Study the drawing (mm; zero at the part's minimum x, y, z) and answer. A direction names the side the tool comes from. Give positions to 0.01 mm unless a question says otherwise; leave off trailing zeros. Loops run counter-clockwise (first coordinate to the right, second up) from the corner with the lowest first, then second, coordinate; pieces in that order, holes last. Notation, with made-up numbers: M 81,15.5 L 135,15.5 A26 cw 135,41.5 Z; hole C 43.5,-24.75 d10. An arc over 180 degrees is marked long. Return JSON: item names as keys, results as strings.
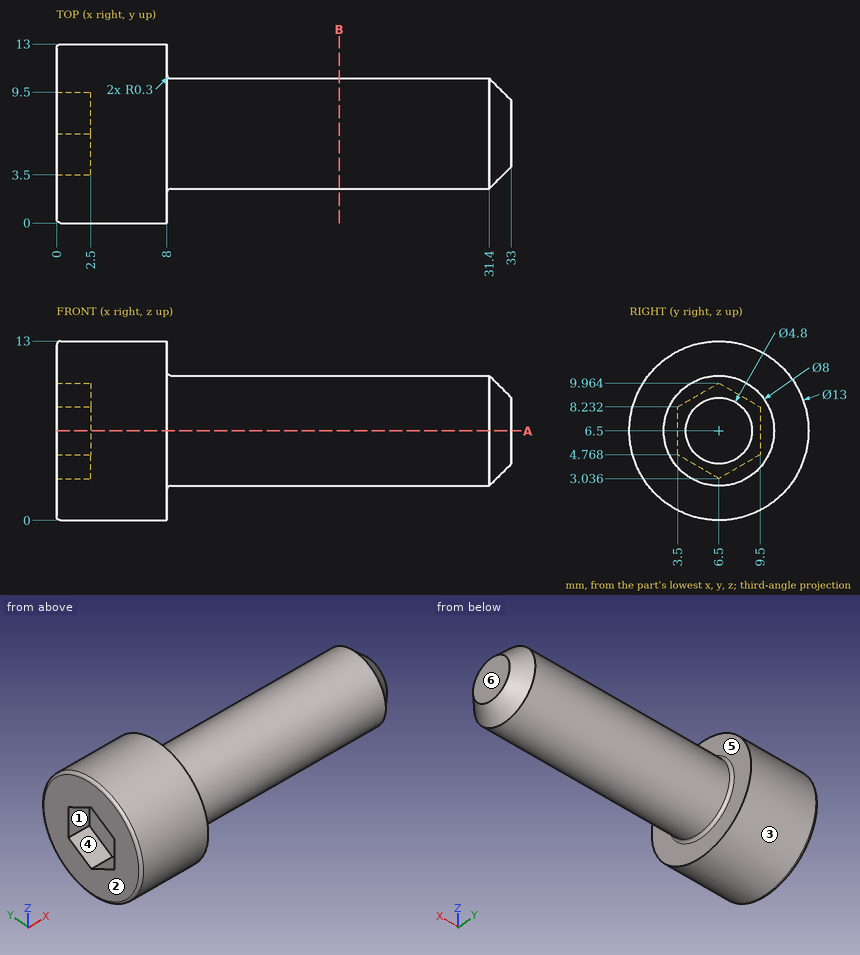
(1) Given pin 1 (2 mm diameter, centred on y = 6, z = 1.5, fed in from -X); pin 2 (1.5 mm diameter, centred on y = 9.5, z = 2.5, fed in from +X); pin 3 (1.8 mm diameter, centred on y = 7, z = 5, fed in from -X); pin 4 (4 mm diameter, centred on x = 29.5, y = 11.5, fed in from +Z), each flat-ended and moving along its own axis, determine where each tip first touches the part or whether it passes through.
Values follow:
{"pin 1": "x = 0", "pin 2": "x = 8", "pin 3": "x = 2.5", "pin 4": "z = 9.15"}
(2) The part is cut by section A-A (z = 6.5). Determine the outline of the cut face in (x, y).
Values follow:
{"outline": "M 0,0.3 A0.3 ccw 0.3,0 L 8,0 L 8,2.2 A0.3 cw 8.3,2.5 L 31.4,2.5 L 33,4.1 L 33,8.9 L 31.4,10.5 L 8.3,10.5 A0.3 cw 8,10.8 L 8,13 L 0.3,13 A0.3 ccw 0,12.7 L 0,9.5 L 2.5,9.5 L 2.5,3.5 L 0,3.5 Z"}
(3) Straight lines are drawn through the part: line 1 along Z through (x, y) = (18, 6.25); line 2 along Y through (x, z) = (13.5, 4.5); line 3 along X through (y, z) = (5.75, 6.75). For each, find the intervals that lie inside material, in ascending order.
Values follow:
{"line 1": "2.51 to 10.49", "line 2": "3.04 to 9.96", "line 3": "2.5 to 33"}
(4) The part is cut by section B-B (x = 20.5). Determine the outline of the cut face in (y, z), and give its area (3 significant figures).
Values follow:
{"outline": "C 6.5,6.5 d8", "area": "50.3 mm²"}
(5) A tool of negligible diameter and unlimited length cuts with its end or side. For the marked faces 5 and 6, from which of +Z, -Z, +X, -X, +Y, -Y can it reach the whole face along a straight path? Write none if from no direction.
Values follow:
{"face 5": "+X", "face 6": "+Z, -Z, +X, +Y, -Y"}
(6) Determine the mould class of the marked faces 1, 2, 3 and 4 for opening direction Y: released by +Y, released by -Y, zero draft, split by the parting line, or undercut.
Values follow:
{"face 1": "undercut", "face 2": "zero draft", "face 3": "split by the parting line", "face 4": "undercut"}
